Source: three-view drawing plus pictorial views. Frame: mm from the lowest corner of the part. Give positions to 0.01 mm unless a question says otherwise; leave off trailing zeros. Loops run counter-clockwise (first coordinate to the right, second up) from the corner with the lowest first, then second, coordinate; pieces in that order, holes last.
1. Section C-C, the plane z = 60. Output: boundary loops of the cut face in (x, y).
2. Section D-D, the plane y = 4.25. Output: boundary loops of the cut face in (x, z).
3. Material intervals for line 1 along Z through (x, y) = (20, 4.75); line 2 along X through (y, z) = (7.75, 17); line 3 along Z through (x, y) = (23, 6.5), sorted ascending.
4. Section A-A, the plane x = 20. Output: boundary loops of the cut face in (y, z), then the cut area to 3 significant figures.
5. Section B-B, the plane z = 20. Output: boundary loops of the cut face in (x, y), then the cut area to 3 significant figures.
6. Draft query along Z for the marked faces 1, 2, 3 and 4. Return one class per face: +Z half, -Z half, draft (parallel to the pull), parting line (faces both ways), or undercut.
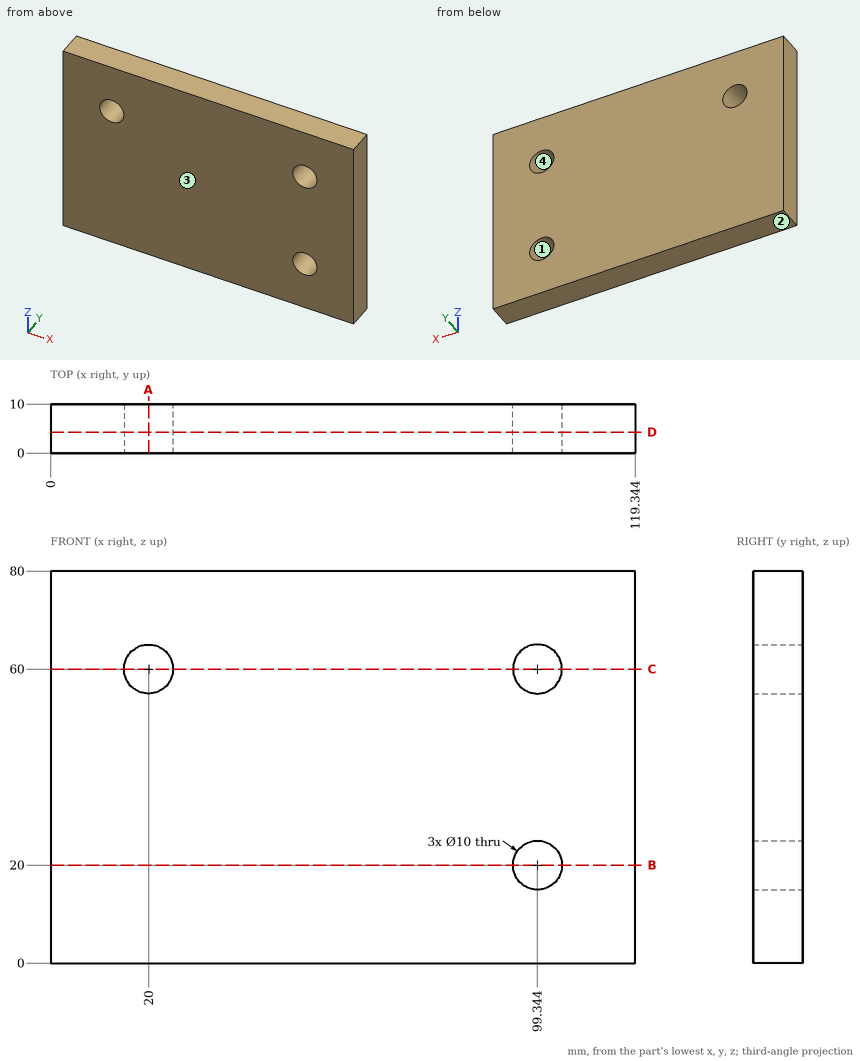
Answers below:
1. outline: (0, 0) - (15, 0) - (15, 10) - (0, 10) - close; (25, 0) - (94.34, 0) - (94.34, 10) - (25, 10) - close; (104.34, 0) - (119.34, 0) - (119.34, 10) - (104.34, 10) - close
2. outline: (0, 0) - (119.34, 0) - (119.34, 80) - (0, 80) - close; hole circle Ø10 at (20, 60); hole circle Ø10 at (99.34, 20); hole circle Ø10 at (99.34, 60)
3. line 1: z = 0 to 55, 65 to 80
3. line 2: x = 0 to 95.34, 103.34 to 119.34
3. line 3: z = 0 to 56, 64 to 80
4. outline: (0, 0) - (10, 0) - (10, 55) - (0, 55) - close; (0, 65) - (10, 65) - (10, 80) - (0, 80) - close
4. area: 700 mm2
5. outline: (0, 0) - (94.34, 0) - (94.34, 10) - (0, 10) - close; (104.34, 0) - (119.34, 0) - (119.34, 10) - (104.34, 10) - close
5. area: 1,090 mm2
6. face 1: undercut
6. face 2: -Z half
6. face 3: draft
6. face 4: undercut
